```python
from build123d import *

# Parameters (mm, degrees)
SKETCH_1_R          = 27.5
EXTRUDE_1_DEPTH     = 56
SKETCH_2_W          = 40
SKETCH_2_H          = 23
EXTRUDE_2_DEPTH     = 2
SKETCH_3_R          = 2.5
CUT_EXTRUDE_1_DEPTH = 2


with BuildPart() as part:
    # 草图1 → 凸台-拉伸1 (new body)
    with BuildSketch(Plane.XY):
        Circle(SKETCH_1_R)
    extrude(amount=EXTRUDE_1_DEPTH)

    # 草图2 → 凸台-拉伸2 (add)
    with BuildSketch(Plane(origin=(0, 0, 0), x_dir=(-1, 0, 0), z_dir=(0, 0, -1))):
        with Locations((0, 30.374586088)):
            Rectangle(SKETCH_2_W, SKETCH_2_H)
    extrude(amount=-EXTRUDE_2_DEPTH)

    # 草图3 → 切除-拉伸1 (cut)
    with BuildSketch(Plane.XY.offset(2)):
        with Locations((0, 34.374586088)):
            Circle(SKETCH_3_R)
        with Locations((-12.5, 34.374586088)):
            Circle(SKETCH_3_R)
        with Locations((12.5, 34.374586088)):
            Circle(SKETCH_3_R)
    extrude(amount=-CUT_EXTRUDE_1_DEPTH, mode=Mode.SUBTRACT)


solid = part.part
```
Work out the finished part from the listing and answer in its coordinate system (mm). A direction names the side the tool comes from. Coordinates: 2 decimals unless noted, no trailing zeros. Order: outer loops, then holes, each group sorted by start corner. A loop starts at its lowest first (then second) coordinate and runs counter-clockwise, first axis right, second up. Notation, with made-up numbers: M 66.5,51.5 L 98.5,51.5 A24 cw 98.5,76.5 Z; hole C 30.5,70 d8. An arc over 180 degrees is marked long. Use CSV: the item, a comma, the result in double quotes.
1) Determine the mould class of faces 1 (the face through (11.958, 31.934, 1.014)), 2 (the face through (0, 41.875, 1)), 3 (the face through (-5.961, -26.846, 27.608)), 4 (the face through (0, 0, 56)) for opening direction Y: released by +Y, released by -Y, zero draft, split by the parting line, or undercut.
Worked out:
face 1,"undercut"
face 2,"released by +Y"
face 3,"split by the parting line"
face 4,"zero draft"
2) Section C-C on z = 45.5 is taken. Write down the section's boundary in (x, y).
Worked out:
outline,"C 0,0 d55"
3) For faces 5 (the face through (-20, 30, 1)), 6 (the face through (20, 30, 1)), 7 (the face through (-0.542, 31.934, 1.014)), determine the directions among +Z, -Z, +X, -X, +Y, -Y from which every point of the face is accessible in a straight line to the end or side of a thin tool.
Worked out:
face 5,"+Z, -Z, -X, +Y"
face 6,"+Z, -Z, +X, +Y"
face 7,"+Z, -Z"
4) Consider line 1 (Y direction, x = 0, z = 1.45); line 2 (Y direction, x = 12, z = 1); line 3 (Z direction, x = -19.5, y = 38.5). Determine where each line is inside the solid, lowest interval first. Write a range as [from, to].
Worked out:
line 1,"y = [-27.5, 31.87], [36.87, 41.87]"
line 2,"y = [-24.74, 31.93], [36.82, 41.87]"
line 3,"z = [0, 2]"
5) Flat-ended cylindrical pins translate along their axes: pin 1 Ø8 at (y, z) = (29, 48) entering from -X; pin 2 Ø4 at (x, y) = (12.5, 34.37) entering from -Z; pin 3 Ø4 at (x, z) = (10, 40) entering from -Y; pin 4 Ø1.5 at (y, z) = (16, 19) entering from -X. Find the tip coordinate at first contact, or state that the pin passes through.
Worked out:
pin 1,"stops at x = -11.46"
pin 2,"passes through"
pin 3,"stops at y = -26.31"
pin 4,"stops at x = -22.88"
6) Section A-A on x = 0 is taken. Write down the section's boundary in (y, z), plus the area to 3 significant figures.
Worked out:
outline,"M -27.5,0 L 31.87,0 L 31.87,2 L 27.5,2 L 27.5,56 L -27.5,56 Z; M 36.87,0 L 41.87,0 L 41.87,2 L 36.87,2 Z"
area,"3,100 mm^2"
7) Section D-D on x = -22 is taken. Write down the section's boundary in (y, z).
Worked out:
outline,"M -16.5,0 L 16.5,0 L 16.5,56 L -16.5,56 Z"
8) Section B-B on y = 26.5 is taken. Write down the section's boundary in (x, z).
Worked out:
outline,"M -20,0 L 20,0 L 20,2 L 7.35,2 L 7.35,56 L -7.35,56 L -7.35,2 L -20,2 Z"
